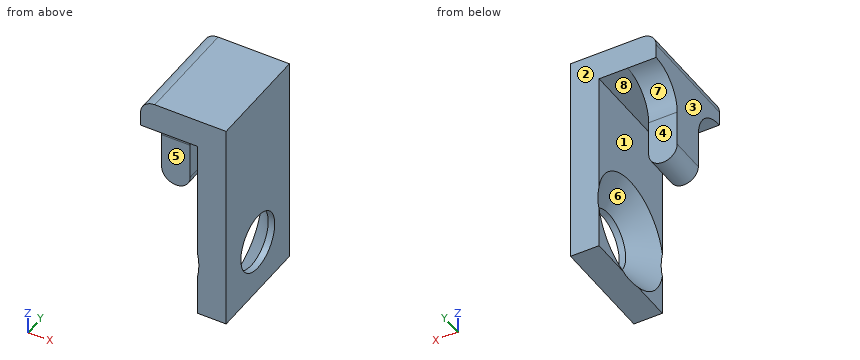
from build123d import *

# Parameters (mm, degrees)
BOSS_EXTRUDE1_DEPTH = 4.7625
CUT_EXTRUDE1_START  = -1.27
CUT_EXTRUDE1_DEPTH  = 6.08


with BuildPart() as part:
    # Sketch1 → Boss-Extrude1 (new body, symmetric)
    with BuildSketch(Plane(origin=(0, 0, 0), x_dir=(1, 0, 0), z_dir=(0, 1, 0))):
        with BuildLine():
            Line((-5.08, -6.985), (-3.81, -6.985))
            Line((-3.81, -6.985), (-3.81, -0.635))
            ThreePointArc((-3.81, -0.635), (-5.08, 0.635), (-6.35, -0.635))
            Line((-6.35, -0.635), (-6.35, -8.255))
            ThreePointArc((-6.35, -8.255), (-5.978025612, -7.356974388), (-5.08, -6.985))
        make_face()
        with BuildLine():
            ThreePointArc((-6.35, -8.255), (-5.978025612, -9.153025612), (-5.08, -9.525))
            ThreePointArc((-5.08, -9.525), (-4.181974388, -9.153025612), (-3.81, -8.255))
            Line((-3.81, -8.255), (-3.81, -6.985))
            Line((-3.81, -6.985), (-5.08, -6.985))
            ThreePointArc((-5.08, -6.985), (-5.978025612, -7.356974388), (-6.35, -8.255))
        make_face()
        with BuildLine():
            Line((-5.08, -9.525), (-1.27, -9.525))
            Line((-1.27, -9.525), (-1.27, -6.985))
            Line((-1.27, -6.985), (-3.81, -6.985))
            Line((-3.81, -6.985), (-3.81, -8.255))
            ThreePointArc((-3.81, -8.255), (-4.181974388, -9.153025612), (-5.08, -9.525))
        make_face()
        with BuildLine():
            Line((-1.27, -6.985), (-1.27, -9.525))
            ThreePointArc((-1.27, -9.525), (0, -8.255), (-1.27, -6.985))
        make_face()
        with BuildLine():
            ThreePointArc((-1.27, -6.985), (0, -8.255), (-1.27, -9.525))
            Line((-1.27, -9.525), (1.27, -9.525))
            Line((1.27, -9.525), (1.27, 9.525))
            Line((1.27, 9.525), (-1.27, 9.525))
            Line((-1.27, 9.525), (-1.27, -6.985))
        make_face()
    extrude(amount=BOSS_EXTRUDE1_DEPTH, both=True)

    # Sketch3 → CSK for #10 Flat Head Machine Screw (100)1 (revolve, cut)
    with BuildSketch(Plane(origin=(-1.27, 0, -4.7625), x_dir=(0, 0, 1), z_dir=(0, 1, 0))):
        Polygon((0, 0), (0, 2.54), (2.5527, 2.54), (2.5527, 1.960808018), (4.8895, 0), align=None)
    revolve(axis=Axis((-7.62, 0, -4.7625), (1, 0, 0)), mode=Mode.SUBTRACT)

    # Sketch4 → Cut-Extrude1 (cut, through all)
    with BuildSketch(Plane(origin=(0, 0, 0), x_dir=(0, 0, -1), z_dir=(1, 0, 0)).offset(CUT_EXTRUDE1_START)):
        with BuildLine():
            Line((0.635, -7.9375), (-3.81, -7.9375))
            ThreePointArc((-3.81, -7.9375), (-6.985, -4.7625), (-3.81, -1.5875))
            Line((-3.81, -1.5875), (0.635, -1.5875))
            ThreePointArc((0.635, -1.5875), (3.81, -4.7625), (0.635, -7.9375))
        make_face()
        with BuildLine():
            Line((0.635, 1.5875), (-3.81, 1.5875))
            ThreePointArc((-3.81, 1.5875), (-6.985, 4.7625), (-3.81, 7.9375))
            Line((-3.81, 7.9375), (0.635, 7.9375))
            ThreePointArc((0.635, 7.9375), (3.81, 4.7625), (0.635, 1.5875))
        make_face()
    extrude(amount=-CUT_EXTRUDE1_DEPTH, mode=Mode.SUBTRACT)


solid = part.part
Input: part model. Units: mm. Frame: model coordinates. Face numbers are marked on the shaded views. A direction names the side the tool comes from. Give positions to 0.01 mm unless a question says otherwise; leave off trailing zeros. Order: outer loops, then holes, each group sorted by start corner. A loop starts at its lowest first (then second) coordinate and runs counter-clockwise, first axis right, second up. Notation, with made-up numbers: (27.5, -25) - (49.5, -25) arc R23 cw to (49.5, 11) - close; hole circle Ø6 at (48, 5.5). An arc over 180 degrees is marked (long way). Answer as a JSON object with one key per item and string values. Group by question number.
Q1. Cut plane A-A, the plane z = 2.5. Output: boundary loops of the cut face in (x, y), then the cut area to 3 significant figures.
Q2. Cut plane C-C, the plane x = -3.5. Output: boundary loops of the cut face in (y, z) (1 decimal), then the cut area to 3 significant figures.
Q3. Line query: probe 1 along Z at (x, y) = (1.1, 0) (3 decimals); probe 2 along X at (y, z) = (-1.5, 1); probe 3 along X at (y, z) = (4.5, 3). Output: solid intervals per line, ascending.
Q4. Cut plane B-B, the plane y = 0. Output: boundary loops of the cut face in (x, z) (3 decimals).
Q5. First-contact query: pin 1 Ø1.3 at (x, z) = (-5, 2) entering from +Y; pin 2 Ø3 at (x, z) = (-5.5, 6) entering from +Y; pin 3 Ø0.8 at (x, y) = (-2.5, -2.5) entering from -Z (3 decimals); pin 4 Ø1.1 at (y, z) = (3.5, -8.5) entering from -X. Flat tips, straight axial feed; report the tip coordinate or a pass-through.
Q6. Cut plane D-D, the plane z = 6.25. Output: boundary loops of the cut face in (x, y).
Q7. Set-up query: the marked faces 1, 2, 3, 4 and 5. Return all of +Z, -Z, +X, -X, +Y, -Y with unobstructed straight access to the full face (end or side cutting, diameter ignored); none if empty.
Q8. Mould query, pull axis Y, two halves, no side actions, for the marked faces 6, 7 and 8. Classes: pulls with the +Y half, pulls with the -Y half, needs draft (parallel to the pull), parting line crosses it, or undercut.
Results:
{
 "1": {"outline": "(-6.35, -1.59) - (-3.81, -1.59) - (-3.81, 1.59) - (-6.35, 1.59) - close; (-1.27, -4.76) - (1.27, -4.76) - (1.27, 4.76) - (-1.27, 4.76) - close", "area": "32.3 mm^2"},
 "2": {"outline": "(-4.8, 7) - (4.8, 7) - (4.8, 9.5) - (-4.8, 9.5) - close", "area": "24.2 mm^2"},
 "3": {"probe 1": "-9.525 to -7.315, -2.21 to 9.525", "probe 2": "-6.35 to -3.81, -1.27 to 1.27", "probe 3": "-1.27 to 1.27"},
 "4": {"outline": "(-6.35, 0.635) arc R1.27 ccw to (-3.81, 0.635) - (-3.81, 6.985) - (-1.27, 6.985) - (-1.27, 0.127) - (0.691, -2.21) - (1.27, -2.21) - (1.27, 9.525) - (-5.08, 9.525) arc R1.27 ccw to (-6.35, 8.255) - close; (-1.163, -9.525) - (1.27, -9.525) - (1.27, -7.315) - (0.691, -7.315) - close"},
 "5": {"pin 1": "y = 1.59", "pin 2": "y = 4.76", "pin 3": "z = 6.985", "pin 4": "x = -1.27"},
 "6": {"outline": "(-6.35, -2.73) - (-3.81, -2.73) - (-3.81, 2.73) - (-6.35, 2.73) - close; (-1.27, -4.76) - (1.27, -4.76) - (1.27, 4.76) - (-1.27, 4.76) - close"},
 "7": {"face 1": "-Z, +Y, -Y", "face 2": "+Z, -Z, +X, -X, +Y", "face 3": "+Z, -Z, -X, +Y, -Y", "face 4": "-Z, -X, +Y", "face 5": "-Z, -X, -Y"},
 "8": {"face 6": "undercut", "face 7": "pulls with the +Y half", "face 8": "needs draft"}
}
